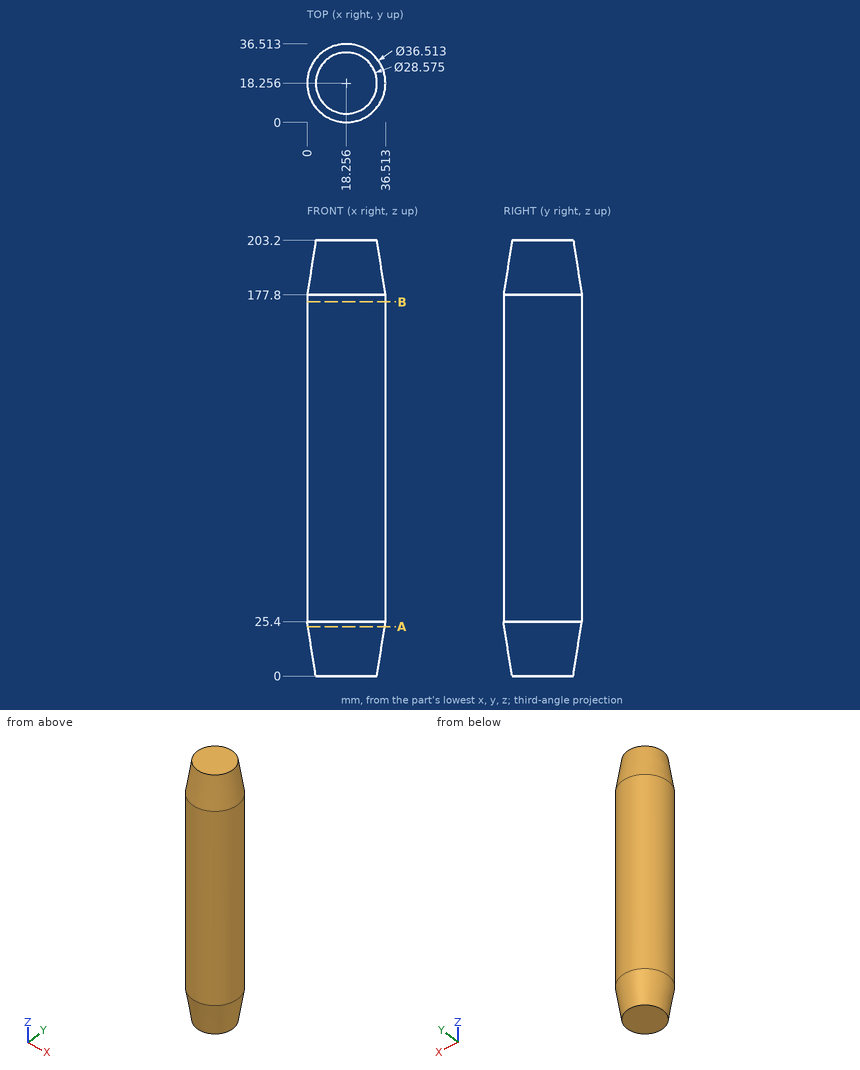
Drawing for the job (mm, zero at the part's lowest x, y, z). Round coordinates to 2 decimals unless told otherwise and drop trailing zeros. Loops run counter-clockwise (first coordinate to the right, second up) from the corner with the lowest first, then second, coordinate; pieces in that order, holes last. Notation, with made-up numbers: (-5, -25) -> (54, -25) arc R22 ccw to (54, 1) -> close; hole circle Ø5 at (-2, -4.75). An arc over 180 degrees is marked (long way). Answer as CSV lines item,"result". Start each with the question number.
1) Slice it at B-B (z = 174.5). List the corners of the cut face in (x, y).
2) Pin check, flat tips, straight feed: P1, Ø5, axis at y = 12, z = 63.5, coming from the +X side; P2, Ø2, axis at x = 10, z = 35.5, coming from the +Y side; P3, Ø4, axis at x = 19.5, z = 94.5, coming from the -Y side. Stop position of each tip, or through.
3) Probe line 1 along Y through (x, z) = (19.5, 138.5); line 2 along Y through (x, z) = (16, 158); line 3 along X through (y, z) = (11, 79.5) (1 decimal). List the from-to ranges inside material, lowest first.
4) Slice it at A-A (z = 23). List the corners of the cut face in (x, y), plus the area to 3 significant figures.
Filled in:
1,outline,"circle Ø36.51 at (18.26, 18.26)"
2,P1,"stops at x = 36.12"
2,P2,"stops at y = 35.01"
2,P3,"stops at y = 0"
3,line 1,"y = 0.04 to 36.47"
3,line 2,"y = 0.14 to 36.37"
3,line 3,"x = 1.5 to 35"
4,outline,"circle Ø35.76 at (18.26, 18.26)"
4,area,"1,000 mm2"
